from build123d import *

# Parameters (mm, degrees)
EXTRUDE_1_DEPTH      = 2
EXTRUDE_1_DEPTH_BACK = 1
SKETCH_1_W           = 31.2
SKETCH_1_H           = 24
EXTRUDE_2_DEPTH      = 36
EXTRUDE_2_DEPTH_BACK = 3
SKETCH_2_W           = 31.2
SKETCH_2_H           = 4
SKETCH_3_R           = 1.4
EXTRUDE_3_DEPTH      = 3
SKETCH_4_R           = 1.4
CUT_EXTRUDE_1_DEPTH  = 8
SKETCH_5_W           = 17
SKETCH_5_H           = 1
CUT_EXTRUDE_2_DEPTH  = 31.2
CUT_EXTRUDE_3_DEPTH  = 31.2
EXTRUDE_START        = 2
SKETCH_7_R           = 1.4
EXTRUDE_4_DEPTH      = 2
EXTRUDE_5_DEPTH      = 10
EXTRUDE_5_DEPTH_BACK = 10
CUT_EXTRUDE_4_DEPTH  = 10


with BuildPart() as part:
    # 草图1 → 凸台-拉伸1 (new, two sides: drawn at the far end of the back side and taken through both)
    with BuildSketch(Plane.XY.offset(-EXTRUDE_1_DEPTH_BACK)):
        Rectangle(SKETCH_1_W, SKETCH_1_H)
    extrude(amount=EXTRUDE_1_DEPTH + EXTRUDE_1_DEPTH_BACK)

    # 草图2 → 凸台-拉伸2 (add, two sides: drawn at the far end of the back side and taken through both)
    with BuildSketch(Plane.XY.offset(2).offset(-EXTRUDE_2_DEPTH_BACK)):
        with Locations((0, 14)):
            Rectangle(SKETCH_2_W, SKETCH_2_H)
        with Locations((0, -14)):
            Rectangle(SKETCH_2_W, SKETCH_2_H)
    extrude(amount=EXTRUDE_2_DEPTH + EXTRUDE_2_DEPTH_BACK)

    # 草图3 → 凸台-拉伸3 (add)
    # profile 1 of 2: a face of its own
    with BuildSketch(Plane.ZY.offset(15.6)):
        Polygon((38, 16), (31, 16), (22.152932489, 16), (32.310715372, 6), (38, 6), align=None)
        with Locations((34, 9)):
            Circle(SKETCH_3_R, mode=Mode.SUBTRACT)
    # profile 2 of 2: a face of its own
    with BuildSketch(Plane.ZY.offset(15.6)):
        Polygon((38, -16), (38, -6), (32.310715372, -6), (22.152932489, -16), (31, -16), align=None)
        with Locations(Location((34, -9, 0), (0, 0, 180))):
            Circle(SKETCH_3_R, mode=Mode.SUBTRACT)
    extrude_3 = extrude(amount=EXTRUDE_3_DEPTH)

    # 草图4 → 切除-拉伸1 (cut)
    with BuildSketch(Plane(origin=(0, 0, -1), x_dir=(-1, 0, 0), z_dir=(0, 0, -1))):
        with Locations((13.6, -14)):
            Circle(SKETCH_4_R)
        with Locations(Location((13.6, 14, 0), (0, 0, 180))):
            Circle(SKETCH_4_R)
        with Locations(Location((-13.6, -14, 0), (0, 0, 180))):
            Circle(SKETCH_4_R)
        with Locations((-13.6, 14)):
            Circle(SKETCH_4_R)
    extrude(amount=-CUT_EXTRUDE_1_DEPTH, mode=Mode.SUBTRACT)

    # 镜向1: 凸台-拉伸3 across plane
    add(extrude_3.mirror(Plane(origin=(0, 0, 0), x_dir=(0, 0, 1), z_dir=(1, 0, 0))))

    # 草图5 → 切除-拉伸2 (cut)
    with BuildSketch(Plane.ZY.offset(15.6)):
        with Locations((27.5, 12.5)):
            Rectangle(SKETCH_5_W, SKETCH_5_H)
        with Locations((27.5, -12.5)):
            Rectangle(SKETCH_5_W, SKETCH_5_H)
    extrude(amount=-CUT_EXTRUDE_2_DEPTH, mode=Mode.SUBTRACT)

    # 草图6 → 切除-拉伸3 (cut)
    with BuildSketch(Plane.ZY.offset(15.6)):
        Polygon((1.3, 0), (1.5, 12), (2, 12), (2, -12), (1.5, -12), align=None)
    extrude(amount=-CUT_EXTRUDE_3_DEPTH, mode=Mode.SUBTRACT)

    # 草图7 → 凸台-拉伸4 (add)
    with BuildSketch(Plane(origin=(0, 0, -1), x_dir=(-1, 0, 0), z_dir=(0, 0, -1)).offset(EXTRUDE_START)):
        Polygon((-15.6, -16), (-15.6, 16), (-15.6, 36), (15.6, 36), (15.6, 16), (15.6, -16), (15.6, -36), (-15.6, -36), align=None)
        with Locations((-13.6, -14)):
            Circle(SKETCH_7_R, mode=Mode.SUBTRACT)
        with Locations((-13.6, 14)):
            Circle(SKETCH_7_R, mode=Mode.SUBTRACT)
        with Locations((13.6, 14)):
            Circle(SKETCH_7_R, mode=Mode.SUBTRACT)
        with Locations((13.6, -14)):
            Circle(SKETCH_7_R, mode=Mode.SUBTRACT)
    extrude(amount=-EXTRUDE_4_DEPTH)

    # 草图8 → 凸台-拉伸5 (add, two sides: drawn at the far end of the back side and taken through both)
    with BuildSketch(Plane(origin=(0, 0, 0), x_dir=(0, 0, -1), z_dir=(1, 0, 0)).offset(-EXTRUDE_5_DEPTH_BACK)):
        Polygon((6.193279754, 21.718771198), (10.887995382, 30.548247127), (3, 30.548247127), (3, 5.223875299), (13, 5.223875299), (13, 5.552438043), (3.15192247, 7.288919819), (4.992593153, 17.727882001), (14.840670683, 15.991400225), (15.022755683, 17.024055571), align=None)
        Polygon((10.887995382, -30.548247127), (3, -30.548247127), (3, -5.223875299), (13, -5.223875299), (13, -5.552438043), (3.15192247, -7.288919819), (4.992593153, -17.727882001), (14.840670683, -15.991400225), (15.022755683, -17.024055571), (6.193279754, -21.718771198), align=None)
    extrude(amount=EXTRUDE_5_DEPTH + EXTRUDE_5_DEPTH_BACK)

    # 草图9 → 切除-拉伸4 (cut)
    with BuildSketch(Plane(origin=(0, 0, -3), x_dir=(-1, 0, 0), z_dir=(0, 0, -1))):
        Polygon((15.6, 36), (-10, 36), (-15.6, 36), (-15.6, 30.548247127), (-10, 30.548247127), (15.6, 30.548247127), align=None)
        Polygon((15.6, -36), (-10, -36), (-15.6, -36), (-15.6, -30.548247127), (-10, -30.548247127), (15.6, -30.548247127), align=None)
    extrude(amount=-CUT_EXTRUDE_4_DEPTH, mode=Mode.SUBTRACT)


solid = part.part
Source: CAD feature listing. Evaluate the final solid. Frame: model axes, mm. A direction names the side the tool comes from. Give positions to 0.01 mm unless a question says otherwise; leave off trailing zeros. Write each loop counter-clockwise with the first axis right and the second up, starting at its lowest first coordinate (ties: lowest second). Pieces come first, ordered by that corner, then holes. Notation, with made-up numbers: M -5.5,89.25 L -1.5,89.25 A8 cw -1.5,99.25 Z; hole C 16,29.25 d6. An arc over 180 degrees is marked long. Answer as a JSON object with one key per item and string values.
Q1. Access query for faces 4 (the face through (-15.6, 10.3, 32.9)), 5 (the face through (0, 23, -1)), 6 (the face through (-0.14, -6.41, -8.14)), 7 (the face through (17.08, 11.07, 27.16)), 8 (the face through (0, 12, 37)). Directions: +Z, -Z, +X, -X, +Y, -Y. A direction counts if a zero-diameter tool reaches every point of the face in a straight line with its end or side. Return the directions, or none.
Geometry check:
{"face 4": "none", "face 5": "+Z, +X, -X, +Y", "face 6": "-Z, +X, -X", "face 7": "-Z, +X", "face 8": "+Z"}
Q2. Cut plane A-A, the plane z = 12. Return the cut outline in (x, y).
Geometry check:
{"outline": "M -15.6,-16 L 15.6,-16 L 15.6,-12 L -15.6,-12 Z; M -15.6,12 L 15.6,12 L 15.6,16 L -15.6,16 Z"}
Q3. Mould query, pull axis Y, two halves, no side actions, for faces 1 (the face through (10, 20, -6)), 2 (the face through (-14, 14, 7)), 3 (the face through (0, 30.548, -5)). Classes: +Y half, -Y half, draft (parallel to the pull), parting line (faces both ways), or undercut.
Geometry check:
{"face 1": "draft", "face 2": "undercut", "face 3": "+Y half"}
Q4. Cut plane C-C, the plane z = 34.5. Count the separate pieces of the cut face and the enclosed holes in it, then the cut area to 3 significant figures.
Geometry check:
{"separate pieces": "6", "enclosed holes": "0", "area": "276 mm^2"}
Q5. Contact query for flat-ended pins moving along their axis: P1, Ø1.5, axis at x = -17.5, z = 35.5, coming from the +Y side; P2, Ø0.9, axis at x = 17.5, z = 35, coming from the -Y side; P3, Ø4, axis at x = -1, y = 7.5, coming from the -Z side. Output: stop coordinate, or through.
Geometry check:
{"P1": "stops at y = 16", "P2": "stops at y = -16", "P3": "stops at z = -13"}
Q6. Cut plane D-D, the plane y = -9. Return the cut outline in (x, z), then the cut area to 3 significant figures.
Geometry check:
{"outline": "M -18.6,29.26 L -15.6,29.26 L -15.6,32.6 L -18.6,32.6 Z; M -18.6,35.4 L -15.6,35.4 L -15.6,38 L -18.6,38 Z; M -15.6,-3 L -10,-3 L -10,-3.45 L 10,-3.45 L 10,-3 L 15.6,-3 L 15.6,1.45 L -15.6,1.45 Z; M 15.6,29.26 L 18.6,29.26 L 18.6,32.6 L 15.6,32.6 Z; M 15.6,35.4 L 18.6,35.4 L 18.6,38 L 15.6,38 Z", "area": "184 mm^2"}
Q7. Ray query, line 1 along Y through (x, z) = (13.6, 0.25); line 2 along Y through (x, z) = (-16.65, 34); line 3 along Y through (x, z) = (8.5, 34). Return the intervals inside material, ascending.
Geometry check:
{"line 1": "y = -16 to -15.4, -12.6 to 12.6, 15.4 to 16", "line 2": "y = -16 to -10.4, -7.6 to -6, 6 to 7.6, 10.4 to 16", "line 3": "y = -16 to -13, 13 to 16"}
